Autodesk Inventor part; units mm, degrees
ref_plane "Work Plane1" through (220, 0, 0) normal (0, 0, -1) x (-1, 0, 0)
ref_plane "YZ Plane" through (0, 0, 0) normal (1, 0, 0) x (0, 1, 0)
ref_plane "XZ Plane" through (0, 0, 0) normal (0, 1, 0) x (-1, 0, 0)
sketch "Sketch1" plane through (0, 0, 0) normal (0, 1, 0) x (-1, 0, 0)
  line L0 (-220, 0) -> (220, 0) construction
  line L1 (-190, -30) -> (190, -30)
  line L2 (190, 30) -> (-190, 30)
  arc A0 (-190, 30) -> (-190, -30) centre (-190, 0) ccw
  arc A1 (190, -30) -> (190, 30) centre (190, 0) ccw
  point P0 (0, 0)
  point P1 (0, 0)
  dimension "d0" = 380
  dimension "d1" = 60
ref_plane "Work Plane1" through (220, 0, 0) normal (0, 0, -1) x (-1, 0, 0)
sketch "Sketch2" plane through (220, 0, 0) normal (0, 0, -1) x (-1, 0, 0)
  line L0 (0, 120) -> (-2, 120)
  line L1 (-2, 120) -> (-2, -120)
  line L2 (-2, -120) -> (0, -120)
  line L3 (0, -120) -> (0, 120)
  line L4 (0, 120) -> (-2, -120) construction
  line L5 (-2, 120) -> (0, -120) construction
  point P0 (220, 0)
  point P1 (-1, 0)
  point P2 (-1, -120)
  point P3 (-1, 120)
  point P4 (0, 0)
  point P5 (-2, 0)
  point P6 (0, 0)
  dimension "d2" = 240
  dimension "d3" = 2
sweep "Sweep1" add profiles "Sketch2" path "Sketch1"
properties part number "HCMUTE-CDT23-BELT_PHAN_LOAI" material "PVC, Unplasticized"
For this review, take the finished solid that the model builds, in its own axes (mm). A direction names the side the tool comes from. Coordinates: 2 decimals unless noted, no trailing zeros. Order: outer loops, then holes, each group sorted by start corner. A loop starts at its lowest first (then second) coordinate and runs counter-clockwise, first axis right, second up. Notation, with made-up numbers: (53.5, -32.5) - (84.5, -32.5) arc R18 ccw to (84.5, -3.5) - close; hole circle Ø3 at (1.5, 1). An arc over 180 degrees is marked (long way). Answer as a JSON object with one key per item and string values. Group by question number.
1. For faces 1 (the cylindrical face through (-219.993, 1.68, -0.66)), 2 (the flat face through (-3, 2, -32)), list the 3-axis set-ups (+Z, -Z, +X, -X, +Y, -Y) from which the entire face can be reached by the end or side of a thin tool; tool diameter is ignored.
2. The part is to be moulded in two halves that separate along X. For faces 3 (the flat face through (-1, 120, -31)), 4 (the flat face through (3, -2, 30)), 5 (the cylindrical face through (221.992, -1.68, -0.704)), say which applies: pulls with the +X half, pulls with the -X half, needs draft (parallel to the pull), parting line crosses it, or undercut.
3. We need section A-A on x = -53. State the section outline as (y, z) points, then the cut area to 3 significant figures.
4. We need section B-B on z = 0. State the section outline as (x, y) points, then the cut area to 3 significant figures.
5. We need section C-C on y = 86.5. State the section outline as (x, z) points.
6. For probe 1 along Z at (x, y) = (-101.5, -94.5); probe 2 along Z at (x, y) = (-195, -68); probe 3 along X at (y, z) = (46, 7.5), list the stretches that pass through material, from the lowest coordinate up.
7. Clearance check with a flat-ended pin moving along its axis: P1, Ø1, axis at y = -38.5, z = -5.5, coming from the -X side. State where the tip first meets the part, or that it passes through.
Final values:
{
 "1": {"face 1": "+Y, -Y", "face 2": "-Z, +X, -X, +Y, -Y"},
 "2": {"face 3": "needs draft", "face 4": "undercut", "face 5": "pulls with the +X half"},
 "3": {"outline": "(-120, -32) - (120, -32) - (120, -30) - (-120, -30) - close; (-120, 30) - (120, 30) - (120, 32) - (-120, 32) - close", "area": "960 mm²"},
 "4": {"outline": "(-222, -120) - (-220, -120) - (-220, 120) - (-222, 120) - close; (220, -120) - (222, -120) - (222, 120) - (220, 120) - close", "area": "960 mm²"},
 "5": {"outline": "(-190, -32) - (190, -32) arc R32 ccw to (190, 32) - (-190, 32) arc R32 ccw to start; hole (-190, -30) - (190, -30) arc R30 ccw to (190, 30) - (-190, 30) arc R30 ccw to start"},
 "6": {"probe 1": "-32 to -30, 30 to 32", "probe 2": "-31.61 to -29.58, 29.58 to 31.61", "probe 3": "-221.11 to -219.05, 219.05 to 221.11"},
 "7": {"P1": "x = -221.61"}
}
